Can you work these out from the model? Positions are in its coordinate system, mm. A direction names the side the tool comes from. Coordinates: 2 decimals unless noted, no trailing zeros. Order: outer loops, then holes, each group sorted by start corner. A loop starts at its lowest first (then second) coordinate and runs counter-clockwise, first axis right, second up. Notation, with made-up numbers: (86.25, 64.25) -> (119.25, 64.25) arc R18 cw to (119.25, 83.25) -> close; hole circle Ø8 at (36, 87). An arc over 180 degrees is marked (long way). Answer as a JSON object with one key per item and string values. Group by question number.
(1) I need wall thicknesses on line 1 (Y direction, x = 463, z = 251); line 2 (Z direction, x = 326.5, y = 78); line 3 (Y direction, x = 354, z = -519.5). Which ranges of each line are inside material? Lowest first, please.
(2) I want a section at C-C, the plane y = 159. List the corners of the cut face in (x, z) for me.
(3) I want a section at D-D, the plane z = -448.5. List the corners of the cut face in (x, y) for me.
(4) I want a section at B-B, the plane x = 286. List the corners of the cut face in (y, z) for me.
(5) Which directions (+Z, -Z, +X, -X, +Y, -Y) give clear straight access to the entire face, cutting with the end or side of a thin tool? Please do faces 1 (the flat face through (279, 200, 125)), 2 (the flat face through (271, -2, -585)), 3 (the flat face through (279, -130, 408)), 4 (the flat face through (279, -200, 125)).
(6) If we mould it in two halves opening along Y, with no side actions, what happens to faces 5 (the flat face through (263, -179, 585)), 6 (the flat face through (279, -170, -235)), 7 (the flat face through (279, 130, 408))? For each: pulls with the +Y half, pulls with the -Y half, needs draft (parallel to the pull), parting line crosses it, or undercut.
(7) For pin 1 (3 mm diameter, centred on x = 159.5, z = 32, fed in from +Y); pin 2 (4 mm diameter, centred on x = 199.5, z = -314, fed in from -Y), each with a flat end and sliding along its axis, tell me the tip position at first contact or that it passes through.
(8) I want a section at A-A, the plane z = 383. List the corners of the cut face in (x, y) for me, plus the area to 3 significant figures.
from build123d import *

# Parameters (mm, degrees)
F1_DEPTH  = 550
F2_W      = 60
F2_H      = 710
F3_DEPTH  = 550.001
F4_W      = 60
F4_H      = 710
F5_DEPTH  = 550.001
F6_W      = 260
F6_H      = 700
F7_DEPTH  = 550.001
F9_DEPTH  = 460.001
F11_DEPTH = 460.001


with BuildPart() as f1:
    # F0 (on Right) → F1 (new body)
    with BuildSketch(Plane.YZ):
        Polygon((-230, 585), (-230, -585), (230, -585), (230, 125), (230, 585), align=None)
    extrude(amount=F1_DEPTH)

    # F2 (on face) → F3 (cut, through all)
    with BuildSketch(Plane.YZ.offset(550)):
        with Locations((-200, -230)):
            Rectangle(F2_W, F2_H)
    extrude(amount=-F3_DEPTH, mode=Mode.SUBTRACT)

    # F4 (on face) → F5 (cut, through all)
    with BuildSketch(Plane.YZ.offset(550)):
        with Locations((200, -230)):
            Rectangle(F4_W, F4_H)
    extrude(amount=-F5_DEPTH, mode=Mode.SUBTRACT)

    # F6 (on face) → F7 (cut, through all)
    with BuildSketch(Plane.YZ.offset(550)):
        with Locations((0, 585)):
            Rectangle(F6_W, F6_H)
    extrude(amount=-F7_DEPTH, mode=Mode.SUBTRACT)

    # F8 (on face) → F9 (cut, through all)
    with BuildSketch(Plane.XZ.offset(230)):
        Polygon((0, 445), (89.0458141333, 585), (0, 585), align=None)
    extrude(amount=-F9_DEPTH, mode=Mode.SUBTRACT)

    # F10 (on face) → F11 (cut, through all)
    with BuildSketch(Plane.XZ.offset(230)):
        Polygon((550, 585), (441.4610564709, 585), (550, 445), align=None)
    extrude(amount=-F11_DEPTH, mode=Mode.SUBTRACT)


solid = f1.part
Computed values:
{
 "1": {"line 1": "y = -230 to -130, 130 to 230", "line 2": "z = -585 to 235", "line 3": "y = -170 to 170"},
 "2": {"outline": "(0, -585) -> (550, -585) -> (550, 445) -> (441.46, 585) -> (89.05, 585) -> (0, 445) -> close"},
 "3": {"outline": "(0, -170) -> (550, -170) -> (550, 170) -> (0, 170) -> close"},
 "4": {"outline": "(-230, 125) -> (-170, 125) -> (-170, -585) -> (170, -585) -> (170, 125) -> (230, 125) -> (230, 585) -> (130, 585) -> (130, 235) -> (-130, 235) -> (-130, 585) -> (-230, 585) -> close"},
 "5": {"face 1": "-Z, +X, -X, +Y", "face 2": "-Z, +X, -X, +Y, -Y", "face 3": "+Z, +X, -X", "face 4": "-Z, +X, -X, -Y"},
 "6": {"face 5": "needs draft", "face 6": "pulls with the -Y half", "face 7": "undercut"},
 "7": {"pin 1": "stops at y = 170", "pin 2": "stops at y = -170"},
 "8": {"outline": "(0, -230) -> (550, -230) -> (550, -130) -> (0, -130) -> close; (0, 130) -> (550, 130) -> (550, 230) -> (0, 230) -> close", "area": "110,000 mm2"}
}
